from build123d import *

# Parameters (mm, degrees)
ESBO_O1_W                                            = 48
ESBO_O1_H                                            = 48
RESSALTO_EXTRUS_O1_DEPTH                             = 6.35
ESBO_O3_R                                            = 6
RESSALTO_EXTRUS_O2_DEPTH                             = 13
CORTE_EXTRUS_O1_START                                = -5
ESBO_O4_R                                            = 6
ESBO_O4_R_2                                          = 2.4
CORTE_EXTRUS_O1_DEPTH                                = 5
CORTE_EXTRUS_O2_START                                = -6.5
ESBO_O5_R                                            = 6
ESBO_O5_R_2                                          = 3.5
CORTE_EXTRUS_O2_DEPTH                                = 6.5
FURO_ROSCADO_DE_M31_D                                = 2.5
FURO_ROSCADO_DE_M31_DEPTH                            = 8.5
FURO_ROSCADO_DE_M31_TIP                              = 0.751075774
ESCAREADO_PARA_PARAFUSO_COM_CABE_A_ESCAR_D           = 3.4
ESCAREADO_PARA_PARAFUSO_COM_CABE_A_ESCAR_DEPTH       = 10.778536948
ESCAREADO_PARA_PARAFUSO_COM_CABE_A_ESCAR_CSINK_D     = 6.3
ESCAREADO_PARA_PARAFUSO_COM_CABE_A_ESCAR_CSINK_ANGLE = 90
ESCAREADO_PARA_PARAFUSO_COM_CABE_A_ESCAR_TIP         = 1.021463052
FURO_ROSCADO_DE_M32_D                                = 2.5
FURO_ROSCADO_DE_M32_DEPTH                            = 9.248924226
FURO_ROSCADO_DE_M32_TIP                              = 0.751075774
CHANFRO4_SIZE                                        = 2
ESBO_O29_R                                           = 4.5
CORTE_EXTRUS_O3_DEPTH                                = 70.115844783
ESCAREADO_PARA_PARAFUSO_COM_CABE_A_E_2_D             = 2.9
ESCAREADO_PARA_PARAFUSO_COM_CABE_A_E_2_CSINK_D       = 5.5
ESCAREADO_PARA_PARAFUSO_COM_CABE_A_E_2_CSINK_ANGLE   = 90
ESBO_O32_R                                           = 17.5
CORTE_EXTRUS_O4_DEPTH                                = 1.6


with BuildPart() as part:
    # Esboço1 → Ressalto-extrusão1 (new body)
    with BuildSketch(Plane.XY):
        with Locations((24, 24)):
            Rectangle(ESBO_O1_W, ESBO_O1_H)
    extrude(amount=RESSALTO_EXTRUS_O1_DEPTH)

    # Esboço3 → Ressalto-extrusão2 (add)
    with BuildSketch(Plane.XY.offset(6.35)):
        with Locations(Location((24, 17.5, 0), (0, 0, 180))):
            Circle(ESBO_O3_R)
    extrude(amount=RESSALTO_EXTRUS_O2_DEPTH)

    # Esboço4 → Corte-extrusão1 (cut)
    with BuildSketch(Plane.XY.offset(19.35).offset(CORTE_EXTRUS_O1_START)):
        with Locations(Location((24, 17.5, 0), (0, 0, 180))):
            Circle(ESBO_O4_R)
        with Locations((24, 17.5)):
            Circle(ESBO_O4_R_2, mode=Mode.SUBTRACT)
    extrude(amount=CORTE_EXTRUS_O1_DEPTH, mode=Mode.SUBTRACT)

    # Esboço5 → Corte-extrusão2 (cut)
    with BuildSketch(Plane.XY.offset(14.35).offset(CORTE_EXTRUS_O2_START)):
        with Locations(Location((24, 17.5, 0), (0, 0, 180))):
            Circle(ESBO_O5_R)
        with Locations((24, 17.5)):
            Circle(ESBO_O5_R_2, mode=Mode.SUBTRACT)
    extrude(amount=CORTE_EXTRUS_O2_DEPTH, mode=Mode.SUBTRACT)

    # Furo roscado de M31
    with Locations(Plane(origin=(24, 17.5, 19.35), x_dir=(1, 0, 0), z_dir=(0, 0, 1))):
        with Locations((0, 0)):
            Hole(FURO_ROSCADO_DE_M31_D / 2, depth=FURO_ROSCADO_DE_M31_DEPTH)
            with Locations((0, 0, -(FURO_ROSCADO_DE_M31_DEPTH + FURO_ROSCADO_DE_M31_TIP / 2))):  # 118° drill point
                Cone(0, FURO_ROSCADO_DE_M31_D / 2, FURO_ROSCADO_DE_M31_TIP, mode=Mode.SUBTRACT)

    # Escareado para parafuso com cabe_a escar
    with Locations(Plane(origin=(44.825, 34, 6.35), x_dir=(1, 0, 0), z_dir=(0, 0, 1))):
        with Locations((0, 0), (-41.65, 0)):
            CounterSinkHole(ESCAREADO_PARA_PARAFUSO_COM_CABE_A_ESCAR_D / 2, ESCAREADO_PARA_PARAFUSO_COM_CABE_A_ESCAR_CSINK_D / 2, depth=ESCAREADO_PARA_PARAFUSO_COM_CABE_A_ESCAR_DEPTH, counter_sink_angle=ESCAREADO_PARA_PARAFUSO_COM_CABE_A_ESCAR_CSINK_ANGLE)
            with Locations((0, 0, -(ESCAREADO_PARA_PARAFUSO_COM_CABE_A_ESCAR_DEPTH + ESCAREADO_PARA_PARAFUSO_COM_CABE_A_ESCAR_TIP / 2))):  # 118° drill point
                Cone(0, ESCAREADO_PARA_PARAFUSO_COM_CABE_A_ESCAR_D / 2, ESCAREADO_PARA_PARAFUSO_COM_CABE_A_ESCAR_TIP, mode=Mode.SUBTRACT)

    # Furo roscado de M32
    with Locations(Plane(origin=(3.175, 0, 3.175), x_dir=(0, 0, -1), z_dir=(0, -1, 0))):
        with Locations((0, 0), (0, 41.65)):
            Hole(FURO_ROSCADO_DE_M32_D / 2, depth=FURO_ROSCADO_DE_M32_DEPTH)
            with Locations((0, 0, -(FURO_ROSCADO_DE_M32_DEPTH + FURO_ROSCADO_DE_M32_TIP / 2))):  # 118° drill point
                Cone(0, FURO_ROSCADO_DE_M32_D / 2, FURO_ROSCADO_DE_M32_TIP, mode=Mode.SUBTRACT)

    # Chanfro4
    # the kernel refuses this chamfer: 2 mm, written as the material it takes off along each edge
    with BuildSketch(Plane(origin=(24, 17.5, 7.85), x_dir=(-1, 0, 0), z_dir=(0, 1, 0))) as chanfro4_piece_1_section:
        Polygon((6, -CHANFRO4_SIZE), (6 - CHANFRO4_SIZE, 0), (6, 0), align=None)
    chanfro4_piece_1 = revolve(axis=Axis((24, 17.5, 7.85), (0, 0, 1)), mode=Mode.PRIVATE)
    chanfro4_piece_1 = split(chanfro4_piece_1, bisect_by=Plane(origin=(28.750537315, 17.5, 6.35), z_dir=(0, 0, 1)), keep=Keep.TOP, mode=Mode.PRIVATE)
    add(chanfro4_piece_1, mode=Mode.SUBTRACT)

    # Esboço29 → Corte-extrusão3 (cut, through all)
    with BuildSketch(Plane.XY.offset(6.35)):
        with Locations((24, 29)):
            Circle(ESBO_O29_R)
    extrude(amount=-CORTE_EXTRUS_O3_DEPTH, mode=Mode.SUBTRACT)

    # Escareado para parafuso com cabe_a e 2 (through all)
    with Locations(Plane(origin=(12.308657049, 22.25, 6.35), x_dir=(1, 0, 0), z_dir=(0, 0, 1))):
        with Locations((0, 0), (23.382685902, 0), (11.691342951, 20.25)):
            CounterSinkHole(ESCAREADO_PARA_PARAFUSO_COM_CABE_A_E_2_D / 2, ESCAREADO_PARA_PARAFUSO_COM_CABE_A_E_2_CSINK_D / 2, counter_sink_angle=ESCAREADO_PARA_PARAFUSO_COM_CABE_A_E_2_CSINK_ANGLE)

    # Esboço32 → Corte-extrusão4 (cut)
    with BuildSketch(Plane(origin=(0, 0, 0), x_dir=(-1, 0, 0), z_dir=(0, 0, -1))):
        with Locations((-24, 29)):
            Circle(ESBO_O32_R)
    extrude(amount=-CORTE_EXTRUS_O4_DEPTH, mode=Mode.SUBTRACT)


solid = part.part
Model file for the job. Use its own axes, mm. A direction names the side the tool comes from. Give positions to 0.01 mm unless a question says otherwise; leave off trailing zeros. Order: outer loops, then holes, each group sorted by start corner. A loop starts at its lowest first (then second) coordinate and runs counter-clockwise, first axis right, second up. Notation, with made-up numbers: (46.5, 56.25) -> (82.5, 56.25) arc R19 ccw to (82.5, 63.25) -> close; hole circle Ø7 at (59.5, 57.5). An arc over 180 degrees is marked (long way). Use CSV: the item, a comma, the result in double quotes.
1. Band-saw the part on D-D, the plane x = 17.5. Give the cut face in (y, z), then the cut area to 3 significant figures.
Outcome:
outline,"(0, 0) -> (12.75, 0) -> (12.75, 1.6) -> (45.25, 1.6) -> (45.25, 0) -> (48, 0) -> (48, 6.35) -> (0, 6.35) -> close"
area,"253 mm²"
2. Drill centre lines: line 1 along X through (y, z) = (22.25, 4.25); line 2 along Y through (x, z) = (24, 4.85); line 3 along Y through (x, z) = (24, 15). Where is each one in solid material? Low to high. Write a range as from..to.
Outcome:
line 1,"0..10.86, 13.76..34.24, 37.14..48"
line 2,"0..24.5, 33.5..41.05, 43.95..48"
line 3,"15.1..16.25, 18.75..19.9"
3. Band-saw the part on C-C, the plane y = 39. Give the cut face in (x, z).
Outcome:
outline,"(0, 0) -> (9.64, 0) -> (9.64, 1.6) -> (38.36, 1.6) -> (38.36, 0) -> (48, 0) -> (48, 6.35) -> (0, 6.35) -> close"
4. Mould opens along X. For faces 1 (the cylindrical face through (43.255, 33.349, 2.416)), 2 (the flat face through (48, 24, 3)), 3 (the flat face through (23, 19, 19.35)) say: +X half, -X half, draft (parallel to the pull), parting line (faces both ways), or undercut.
Outcome:
face 1,"undercut"
face 2,"+X half"
face 3,"draft"
5. 3-axis set-ups, long thin cutter, end or side, ignore diameter. For faces 4 (the conical face through (3.24, 9.87, 2.97)), 5 (the cylindrical face through (22.845, 17.021, 15.041)), 6 (the cylindrical face through (26.28, 46.35, 0.79)): which of +Z, -Z, +X, -X, +Y, -Y reach the whole face in a straight line?
Outcome:
face 4,"-Y"
face 5,"+Z"
face 6,"-Z"
6. Drop flat-ended pins along their axis: pin 1 (2.5 mm diameter, centred on x = 3.175, y = 34, fed in from -Z); pin 2 (3.5 mm diameter, centred on x = 35.69, y = 22.25, fed in from -Z); pin 3 (14.5 mm diameter, centred on x = 18.5, y = 26, fed in from +Z); pin 4 (11.5 mm diameter, centred on x = 24, y = 29, fed in from +Z). Give the stop position or say it passes through.
Outcome:
pin 1,"through"
pin 2,"z = 1.6"
pin 3,"z = 14.35"
pin 4,"z = 6.35"
7. Band-saw the part on B-B, the plane z = 17. Give the cut face in (x, y).
Outcome:
outline,"circle Ø4.8 at (24, 17.5); hole circle Ø2.5 at (24, 17.5)"
8. Band-saw the part on A-A, the plane y = 29. Give the cut face in (x, z).
Outcome:
outline,"(0, 0) -> (6.5, 0) -> (6.5, 1.6) -> (19.5, 1.6) -> (19.5, 6.35) -> (0, 6.35) -> close; (28.5, 1.6) -> (41.5, 1.6) -> (41.5, 0) -> (48, 0) -> (48, 6.35) -> (28.5, 6.35) -> close"
